```python
from build123d import *

# Parameters (mm, degrees)
SKETCH1_R           = 1.35
SKETCH1_W           = 20
SKETCH1_H           = 40.3
BOSS_EXTRUDE1_DEPTH = 5.9944


with BuildPart() as part:
    # Sketch1 → Boss-Extrude1 (new body)
    with BuildSketch(Plane.XY):
        with BuildLine():
            ThreePointArc((-18.89, 17.61), (-14.426307345, 28.386307345), (-3.65, 32.85))
            Line((-3.65, 32.85), (10, 32.85))
            Line((10, 32.85), (22.7, 32.85))
            Line((22.7, 32.85), (28.6944, 32.85))
            Line((28.6944, 32.85), (28.6944, 20.15))
            Line((28.6944, 20.15), (22.7, 20.15))
            Line((22.7, 20.15), (22.7, 6.35))
            Line((22.7, 6.35), (28.6944, 6.35))
            Line((28.6944, 6.35), (28.6944, 0))
            Line((28.6944, 0), (28.6944, -6.35))
            Line((28.6944, -6.35), (22.7, -6.35))
            Line((22.7, -6.35), (22.7, -20.15))
            Line((22.7, -20.15), (28.6944, -20.15))
            Line((28.6944, -20.15), (28.6944, -32.85))
            Line((28.6944, -32.85), (22.7, -32.85))
            Line((22.7, -32.85), (-3.65, -32.85))
            ThreePointArc((-3.65, -32.85), (-14.426307345, -28.386307345), (-18.89, -17.61))
            Line((-18.89, -17.61), (-18.89, 17.61))
        make_face()
        with Locations((5, 24.5)):
            Circle(SKETCH1_R, mode=Mode.SUBTRACT)
        with Locations((-5, 24.5)):
            Circle(SKETCH1_R, mode=Mode.SUBTRACT)
        with Locations((5, -24.5)):
            Circle(SKETCH1_R, mode=Mode.SUBTRACT)
        with Locations((-5, -24.5)):
            Circle(SKETCH1_R, mode=Mode.SUBTRACT)
        Rectangle(SKETCH1_W, SKETCH1_H, mode=Mode.SUBTRACT)
    extrude(amount=BOSS_EXTRUDE1_DEPTH)


solid = part.part
```
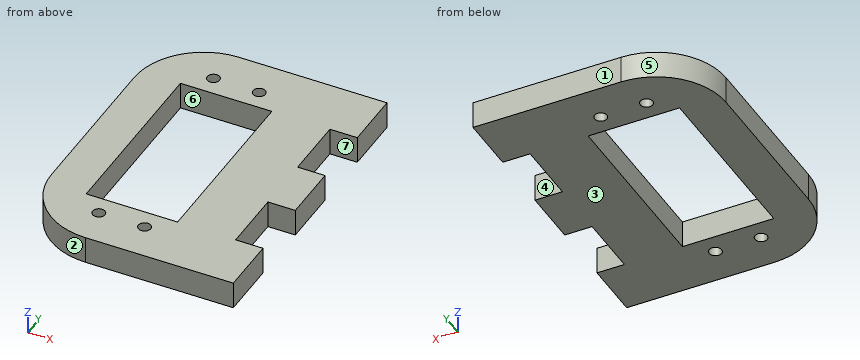
For this review, take the finished solid that the model builds, in its own axes (mm). Face numbers are marked on the shaded views. A direction names the side the tool comes from. Coordinates: 2 decimals unless noted, no trailing zeros. Loops run counter-clockwise (first coordinate to the right, second up) from the corner with the lowest first, then second, coordinate; pieces in that order, holes last.
1. Insertion check: P1, Ø8, axis at x = 5, y = 20, coming from the -Z side; P2, Ø3, axis at y = -16, z = 3, coming from the +X side; P3, Ø2.5, axis at x = -5, y = 24.5, coming from the -Z side; P4, Ø2, axis at y = -21, z = 5, coming from the -X side. Each pin has a flat end and moves straight along its axis. Give the tip position at first contact, or say it passes through.
2. Add section D-D, the plane y = -24.5. Give the boundary of the cut face in (x, z).
3. Add section B-B, the plane y = 9.5. Give the boundary of the cut face in (x, z).
4. Mouldability with a two-part tool opening along Y and no side actions: class the marked faces 1, 2, 3 and 4 as +Y half, -Y half, draft (parallel to the pull), parting line (faces both ways), or undercut.
5. Add section C-C, the plane z = 1.8. Give the boundary of the cut face in (x, y), then the cut area to 3 significant figures.
6. For line 1 (Y direction, x = 26.5, z = 4.4); line 2 (X direction, y = 10.5, z = 3.6); line 3 (Y direction, x = 2, z = 5.15), list the stretches that pass through material, from the lowest coordinate up.
7. For the marked faces 5, 6 and 7, list the 3-axis set-ups (+Z, -Z, +X, -X, +Y, -Y) from which the entire face can be reached by the end or side of a thin tool; tool diameter is ignored.
8. Add section A-A, the plane x = 5. Give the boundary of the cut face in (y, z).
Result:
1. P1: stops at z = 0
1. P2: stops at x = 22.7
1. P3: passes through
1. P4: stops at x = -18.7
2. outline: (-17.24, 0) - (-6.35, 0) - (-6.35, 5.99) - (-17.24, 5.99) - close; (-3.65, 0) - (3.65, 0) - (3.65, 5.99) - (-3.65, 5.99) - close; (6.35, 0) - (28.69, 0) - (28.69, 5.99) - (6.35, 5.99) - close
3. outline: (-18.89, 0) - (-10, 0) - (-10, 5.99) - (-18.89, 5.99) - close; (10, 0) - (22.7, 0) - (22.7, 5.99) - (10, 5.99) - close
4. face 1: +Y half
4. face 2: -Y half
4. face 3: draft
4. face 4: undercut
5. outline: (-18.89, -17.61) arc R15.24 ccw to (-3.65, -32.85) - (28.69, -32.85) - (28.69, -20.15) - (22.7, -20.15) - (22.7, -6.35) - (28.69, -6.35) - (28.69, 6.35) - (22.7, 6.35) - (22.7, 20.15) - (28.69, 20.15) - (28.69, 32.85) - (-3.65, 32.85) arc R15.24 ccw to (-18.89, 17.61) - close; hole (-10, -20.15) - (10, -20.15) - (10, 20.15) - (-10, 20.15) - close; hole circle Ø2.7 at (-5, -24.5); hole circle Ø2.7 at (-5, 24.5); hole circle Ø2.7 at (5, -24.5); hole circle Ø2.7 at (5, 24.5)
5. area: 2,030 mm2
6. line 1: y = -32.85 to -20.15, -6.35 to 6.35, 20.15 to 32.85
6. line 2: x = -18.89 to -10, 10 to 22.7
6. line 3: y = -32.85 to -20.15, 20.15 to 32.85
7. face 5: +Z, -Z, -X, +Y
7. face 6: +Z, -Z
7. face 7: +Z, -Z, +X
8. outline: (-32.85, 0) - (-25.85, 0) - (-25.85, 5.99) - (-32.85, 5.99) - close; (-23.15, 0) - (-20.15, 0) - (-20.15, 5.99) - (-23.15, 5.99) - close; (20.15, 0) - (23.15, 0) - (23.15, 5.99) - (20.15, 5.99) - close; (25.85, 0) - (32.85, 0) - (32.85, 5.99) - (25.85, 5.99) - close
